from build123d import *

# Parameters (mm, degrees)
SKETCH1_W           = 78.74
SKETCH1_H           = 56.388
BOSS_EXTRUDE1_DEPTH = 2.54
FILLET1_R           = 2.54
SKETCH2_R           = 2.54
CUT_EXTRUDE1_DEPTH  = 2.54


with BuildPart() as part:
    # Sketch1 → Boss-Extrude1 (new body)
    with BuildSketch(Plane(origin=(0, 0, 0), x_dir=(1, 0, 0), z_dir=(0, 1, 0))):
        Rectangle(SKETCH1_W, SKETCH1_H)
    extrude(amount=BOSS_EXTRUDE1_DEPTH)

    # Fillet1
    fillet1_edges = [part.edges().sort_by_distance(p)[0] for p in [
        (39.37, 1.27, 28.194),
        (-39.37, 1.27, 28.194),
        (-39.37, 1.27, -28.194),
        (39.37, 1.27, -28.194),
    ]]
    fillet(fillet1_edges, radius=FILLET1_R)

    # Sketch2 → Cut-Extrude1 (cut)
    with BuildSketch(Plane(origin=(0, 2.54, 0), x_dir=(1, 0, 0), z_dir=(0, 1, 0))):
        with Locations(Location((31.75, 20.6375, 0), (0, 0, 270))):
            Circle(SKETCH2_R)
        with Locations(Location((31.75, -20.6375, 0), (0, 0, 270))):
            Circle(SKETCH2_R)
        with Locations(Location((-31.75, -20.6375, 0), (0, 0, 270))):
            Circle(SKETCH2_R)
        with Locations(Location((-31.75, 20.6375, 0), (0, 0, 270))):
            Circle(SKETCH2_R)
        with Locations(Location((-22.225, -20.6375, 0), (0, 0, 270))):
            Circle(SKETCH2_R)
        with Locations(Location((-22.225, 20.6375, 0), (0, 0, 270))):
            Circle(SKETCH2_R)
    extrude(amount=-CUT_EXTRUDE1_DEPTH, mode=Mode.SUBTRACT)


solid = part.part
The model under review builds one solid part; all positions refer to its coordinate system, in mm. Coordinates: 2 decimals unless noted, no trailing zeros. Loops run counter-clockwise (first coordinate to the right, second up) from the corner with the lowest first, then second, coordinate; pieces in that order, holes last. Notation, with made-up numbers: (-2, 0) -> (20, 0) arc R23 ccw to (20, 21) -> close; hole circle Ø4 at (-1.75, 57). An arc over 180 degrees is marked (long way). Use a Markdown table: item, result. Add a question column.
1. Add section A-A on x = -31.75. Write out the cut boundary in (y, z).
2. Add section C-C on x = 30.5. Write out the cut boundary in (y, z), plus the area to 3 significant figures.
3. To check wall thickness, follow line 1 (Z direction, x = -32, y = 2.15); line 2 (Z direction, x = 34, y = 1.2); line 3 (X direction, y = 1.95, z = 21). State the ranges of each line that lie inside material, in increasing order.
4. Draft analysis for pull direction Z (two halves, no side actions). For faces 1 (the face through (-38.646, 1.288, -27.43)), 2 (the face through (-39.37, 1, 0)), 3 (the face through (-29.23, 1.29, 20.31)), 4 (the face through (-1, 1, 28.194)), state which applies: pulls with the +Z half, pulls with the -Z half, needs draft (parallel to the pull), parting line crosses it, or undercut.
5. Add section B-B on y = 0.7. Give the number of separate pieces and of enclosed holes in the cut face, plus the area to 3 significant figures.
Returned:
| question | item | result |
|---|---|---|
| 1 | outline | (0, -28.19) -> (2.54, -28.19) -> (2.54, -23.18) -> (0, -23.18) -> close; (0, -18.1) -> (2.54, -18.1) -> (2.54, 18.1) -> (0, 18.1) -> close; (0, 23.18) -> (2.54, 23.18) -> (2.54, 28.19) -> (0, 28.19) -> close |
| 2 | outline | (0, -28.19) -> (2.54, -28.19) -> (2.54, -22.85) -> (0, -22.85) -> close; (0, -18.43) -> (2.54, -18.43) -> (2.54, 18.43) -> (0, 18.43) -> close; (0, 22.85) -> (2.54, 22.85) -> (2.54, 28.19) -> (0, 28.19) -> close |
| 2 | area | 121 mm² |
| 3 | line 1 | z = -28.19 to -23.17, -18.11 to 18.11, 23.17 to 28.19 |
| 3 | line 2 | z = -28.19 to -21.82, -19.46 to 19.46, 21.82 to 28.19 |
| 3 | line 3 | x = -39.37 to -34.26, -29.24 to -24.74, -19.71 to 29.24, 34.26 to 39.37 |
| 4 | face 1 | pulls with the -Z half |
| 4 | face 2 | needs draft |
| 4 | face 3 | undercut |
| 4 | face 4 | pulls with the +Z half |
| 5 | separate pieces | 1 |
| 5 | enclosed holes | 6 |
| 5 | area | 4,310 mm² |
